```python
from build123d import *

# Parameters (mm, degrees)
BOSS_EXTRUDE1_DEPTH      = 1.5
BOSS_EXTRUDE1_DEPTH_BACK = 1.5
BOSS_EXTRUDE2_START      = 1.5
SKETCH1_3_R              = 1
BOSS_EXTRUDE2_DEPTH      = 2.5
BOSS_EXTRUDE3_START      = -4
SKETCH1_4_R              = 1
BOSS_EXTRUDE3_DEPTH      = 2.5
FILLET1_R                = 2
CUT_EXTRUDE1_DEPTH       = 41.943081007
CUT_EXTRUDE1_DEPTH_BACK  = 41.943081007
FILLET2_R                = 2


with BuildPart() as part:
    # Sketch1 → Boss-Extrude1 (new, two sides: drawn at the far end of the back side and taken through both)
    with BuildSketch(Plane(origin=(0, 0, 0), x_dir=(0, 0, -1), z_dir=(1, 0, 0)).offset(-BOSS_EXTRUDE1_DEPTH_BACK)):
        Polygon((21.723642207, 10.27531536), (14.942385879, 9.950712214), (15.181450651, 4.95643068), (21.962706979, 5.281033826), align=None)
        Polygon((28.504898535, 10.599918506), (21.723642207, 10.27531536), (21.962706979, 5.281033826), (28.743963307, 5.605636972), align=None)
    extrude(amount=BOSS_EXTRUDE1_DEPTH + BOSS_EXTRUDE1_DEPTH_BACK)

    # Sketch1_3 → Boss-Extrude2 (add)
    # profile 1 of 4: a face of its own
    with BuildSketch(Plane(origin=(0, 0, 0), x_dir=(0, 0, -1), z_dir=(1, 0, 0)).offset(BOSS_EXTRUDE2_START)):
        Polygon((14.942385879, 9.950712214), (4.454394659, 9.448676193), (4.693459431, 4.454394659), (15.181450651, 4.95643068), align=None)
        with Locations((7.071067812, 7.071067812)):
            Circle(SKETCH1_3_R, mode=Mode.SUBTRACT)
    # profile 2 of 4: a face of its own
    with BuildSketch(Plane(origin=(0, 0, 0), x_dir=(0, 0, -1), z_dir=(1, 0, 0)).offset(BOSS_EXTRUDE2_START)):
        Polygon((21.723642207, 10.27531536), (14.942385879, 9.950712214), (15.181450651, 4.95643068), (21.962706979, 5.281033826), align=None)
    # profile 3 of 4: a face of its own
    with BuildSketch(Plane(origin=(0, 0, 0), x_dir=(0, 0, -1), z_dir=(1, 0, 0)).offset(BOSS_EXTRUDE2_START)):
        Polygon((28.504898535, 10.599918506), (21.723642207, 10.27531536), (21.962706979, 5.281033826), (28.743963307, 5.605636972), align=None)
    # profile 4 of 4: a face of its own
    with BuildSketch(Plane(origin=(0, 0, 0), x_dir=(0, 0, -1), z_dir=(1, 0, 0)).offset(BOSS_EXTRUDE2_START)):
        Polygon((38.992889755, 11.101954527), (28.504898535, 10.599918506), (28.743963307, 5.605636972), (39.231954527, 6.107672994), align=None)
        with Locations((36.615281374, 8.485281374)):
            Circle(SKETCH1_3_R, mode=Mode.SUBTRACT)
    extrude(amount=BOSS_EXTRUDE2_DEPTH)

    # Sketch1_4 → Boss-Extrude3 (add)
    # profile 1 of 4: a face of its own
    with BuildSketch(Plane(origin=(0, 0, 0), x_dir=(0, 0, -1), z_dir=(1, 0, 0)).offset(BOSS_EXTRUDE3_START)):
        Polygon((14.942385879, 9.950712214), (4.454394659, 9.448676193), (4.693459431, 4.454394659), (15.181450651, 4.95643068), align=None)
        with Locations((7.071067812, 7.071067812)):
            Circle(SKETCH1_4_R, mode=Mode.SUBTRACT)
    # profile 2 of 4: a face of its own
    with BuildSketch(Plane(origin=(0, 0, 0), x_dir=(0, 0, -1), z_dir=(1, 0, 0)).offset(BOSS_EXTRUDE3_START)):
        Polygon((21.723642207, 10.27531536), (14.942385879, 9.950712214), (15.181450651, 4.95643068), (21.962706979, 5.281033826), align=None)
    # profile 3 of 4: a face of its own
    with BuildSketch(Plane(origin=(0, 0, 0), x_dir=(0, 0, -1), z_dir=(1, 0, 0)).offset(BOSS_EXTRUDE3_START)):
        Polygon((28.504898535, 10.599918506), (21.723642207, 10.27531536), (21.962706979, 5.281033826), (28.743963307, 5.605636972), align=None)
    # profile 4 of 4: a face of its own
    with BuildSketch(Plane(origin=(0, 0, 0), x_dir=(0, 0, -1), z_dir=(1, 0, 0)).offset(BOSS_EXTRUDE3_START)):
        Polygon((38.992889755, 11.101954527), (28.504898535, 10.599918506), (28.743963307, 5.605636972), (39.231954527, 6.107672994), align=None)
        with Locations((36.615281374, 8.485281374)):
            Circle(SKETCH1_4_R, mode=Mode.SUBTRACT)
    extrude(amount=BOSS_EXTRUDE3_DEPTH)

    # Fillet1
    fillet1_edges = [part.edges().sort_by_distance(p)[0] for p in [
        (2.75, 11.101954527, -38.992889755),
        (2.75, 9.448676193, -4.454394659),
        (-2.75, 9.448676193, -4.454394659),
        (-2.75, 11.101954527, -38.992889755),
    ]]
    fillet(fillet1_edges, radius=FILLET1_R)

    # Sketch3 → Cut-Extrude1 (cut, two sides: drawn at the far end of the back side and taken through both)
    with BuildSketch(Plane(origin=(0, 0, 0), x_dir=(0, 0, -1), z_dir=(1, 0, 0)).offset(-CUT_EXTRUDE1_DEPTH_BACK)):
        with BuildLine():
            ThreePointArc((6.951535426, 9.568208579), (8.33880017, 9.225796256), (9.311922174, 8.17947736))
            Line((9.311922174, 8.17947736), (34.278801103, 9.37458444))
            ThreePointArc((34.278801103, 9.37458444), (35.147533078, 10.50906865), (36.495748988, 10.982422141))
            Line((36.495748988, 10.982422141), (36.350334975, 14.020253749))
            Line((36.350334975, 14.020253749), (6.806121413, 12.606040186))
            Line((6.806121413, 12.606040186), (6.951535426, 9.568208579))
        make_face()
    extrude(amount=CUT_EXTRUDE1_DEPTH + CUT_EXTRUDE1_DEPTH_BACK, mode=Mode.SUBTRACT)

    # Fillet2
    fillet2_edges = [part.edges().sort_by_distance(p)[0] for p in [
        (2.75, 8.17947736, -9.311922174),
        (-2.75, 9.37458444, -34.278801103),
        (2.75, 9.37458444, -34.278801103),
        (-2.75, 8.17947736, -9.311922174),
    ]]
    fillet(fillet2_edges, radius=FILLET2_R)


solid = part.part
```
For this review, take the finished solid that the model builds, in its own axes (mm). A direction names the side the tool comes from. Coordinates: 2 decimals unless noted, no trailing zeros. Loops run counter-clockwise (first coordinate to the right, second up) from the corner with the lowest first, then second, coordinate; pieces in that order, holes last.
1. Add section A-A, the plane z = -31. Give the boundary of the cut face in (x, y), then the cut area to 3 significant figures.
2. Insertion check: P1, Ø3, axis at x = 1, z = -11.5, coming from the -Y side; P2, Ø3, axis at y = 7.07, z = -7.07, coming from the +X side; P3, Ø1.6, axis at y = 8.49, z = -36.62, coming from the +X side; P4, Ø1, axis at x = -0.5, z = -25.5, coming from the -Y side. Each pin has a flat end and moves straight along its axis. Give the tip position at first contact, or say it passes through.
3. Mouldability with a two-part tool opening along Z and no side actions: class faces 3 (the cylindrical face through (-2.768, 7.914, -7.609)), 4 (the flat face through (1.5, 8, -34)), 5 (the cylindrical face through (2.77, 9.53, -34.01)), 6 (the flat face through (-0.021, 6.729, -15.097)) as +Z half, -Z half, draft (parallel to the pull), parting line (faces both ways), or undercut.
4. For line 1 (X direction, y = 6.5, z = -12); line 2 (Z direction, x = -2.75, y = 7); line 3 (Y direction, x = -2.75, z = -36), list the stretches that pass through material, from the lowest coordinate up.
5. For faces 1 (the flat face through (-0.06, 8.77, -21.64)), 2 (the flat face through (-2.77, 5.97, -4.62)), list the 3-axis set-ups (+Z, -Z, +X, -X, +Y, -Y) from which the entire face can be reached by the end or side of a thin tool; tool diameter is ignored.
6. Add section D-D, the plane z = -18. Give the boundary of the cut face in (x, y), then the cut area to 3 significant figures.
7. Add section B-B, the plane x = -2.5. Give the boundary of the cut face in (y, z), then the cut area to 3 significant figures.
8. Add section C-C, the plane x = 0. Give the boundary of the cut face in (y, z).
Result:
1. outline: (-4, 5.71) - (-1.5, 5.71) - (-1.5, 9.22) - (-4, 9.22) - close; (1.5, 5.71) - (4, 5.71) - (4, 9.22) - (1.5, 9.22) - close
1. area: 17.5 mm2
2. P1: stops at y = 4.71
2. P2: stops at x = 4
2. P3: passes through
2. P4: stops at y = 5.43
3. face 3: undercut
3. face 4: draft
3. face 5: undercut
3. face 6: +Z half
4. line 1: x = -4 to -1.5, 1.5 to 4
4. line 2: z = -39.19 to -8.07, -6.07 to -4.57
4. line 3: y = 5.95 to 7.7, 9.27 to 10.91
5. face 1: +X, -X, +Y
5. face 2: +Z, +X, -X, -Y
6. outline: (-4, 5.09) - (4, 5.09) - (4, 8.6) - (-4, 8.6) - close
6. area: 28.0 mm2
7. outline: (4.45, -4.69) - (6.11, -39.23) - (9.1, -39.09) arc R2 ccw to (11.01, -37) - (10.98, -36.5) arc R2.5 ccw to (10.06, -34.67) arc R2 cw to (9.32, -33.22) - (8.23, -10.37) arc R2 cw to (8.82, -8.85) arc R2.5 ccw to (9.57, -6.95) - (9.54, -6.45) arc R2 ccw to (7.45, -4.55) - close; hole circle Ø2 at (7.07, -7.07); hole circle Ø2 at (8.49, -36.62)
7. area: 126 mm2
8. outline: (4.96, -15.18) - (5.61, -28.74) - (9.1, -28.58) - (8.45, -15.01) - close
